Could you check a few things on this model? Use its own coordinates, in mm. Face numbers are marked on the shaded views. A direction names the side the tool comes from. Give positions to 0.01 mm unless a question says otherwise; leave off trailing zeros. Order: outer loops, then holes, each group sorted by start corner. A loop starts at its lowest first (then second) coordinate and runs counter-clockwise, first axis right, second up.
from build123d import *

# Parameters (mm, degrees)
F2_SIZE = 5
F3_SIZE = 3
F4_SIZE = 1


with BuildPart() as f1:
    # F0 (on Front) → F1 (revolve)
    with BuildSketch(Plane.XZ):
        Polygon((0, 5), (0, 0), (55, 0), (55, 12), (26, 12), (26, 19.5), (4, 19.5), (4, 7.25), (-2, 7.25), (-2, 5), align=None)
    revolve(axis=Axis((27.5, 0, 0), (-1, 0, 0)))

    # F2
    f2_edges = [f1.edges().sort_by_distance(p)[0] for p in [
        (4, 0, -19.5),
    ]]
    chamfer(f2_edges, length=F2_SIZE)

    # F3
    f3_edges = [f1.edges().sort_by_distance(p)[0] for p in [
        (26, 0, -19.5),
        (55, 0, -12),
    ]]
    chamfer(f3_edges, length=F3_SIZE)

    # F4
    f4_edges = [f1.edges().sort_by_distance(p)[0] for p in [
        (-2, 0, -7.25),
    ]]
    chamfer(f4_edges, length=F4_SIZE)


solid = f1.part
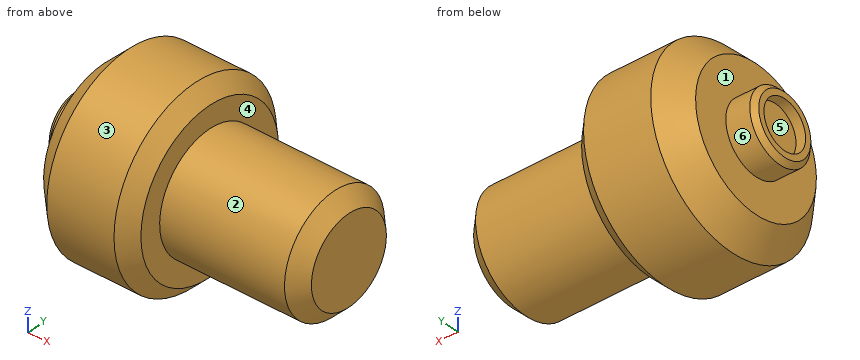
Item 1: For pin 1 (5 mm diameter, centred on y = 0, z = -1.5, fed in from -X); pin 2 (1.5 mm diameter, centred on x = 30, z = 11.5, fed in from -Y); pin 3 (1.5 mm diameter, centred on y = -6.5, z = 15.5, fed in from +X), each with a flat end and sliding along its axis, tell me the tip position at first contact or that it passes through.
Findings:
pin 1: stops at x = 0
pin 2: stops at y = -5.33
pin 3: stops at x = 26
Item 2: Imagine slicing it at A-A on y = 0. List the corners of the cut face in (x, z) for me, then the cut area to 3 significant figures.
Findings:
outline: (-2, -6.25) - (-1, -7.25) - (4, -7.25) - (4, -14.5) - (9, -19.5) - (23, -19.5) - (26, -16.5) - (26, -12) - (52, -12) - (55, -9) - (55, 9) - (52, 12) - (26, 12) - (26, 16.5) - (23, 19.5) - (9, 19.5) - (4, 14.5) - (4, 7.25) - (-1, 7.25) - (-2, 6.25) - (-2, 5) - (0, 5) - (0, -5) - (-2, -5) - close
area: 1,580 mm2
Item 3: Please list where these lines run through material, in increasing order: line 1 along Y through (x, z) = (18.5, 0); line 2 along Y through (x, z) = (-1, 0); line 3 along X through (y, z) = (-3, 12.5).
Findings:
line 1: y = -19.5 to 19.5
line 2: y = -7.25 to -5, 5 to 7.25
line 3: x = 4 to 26
Item 4: Imagine slicing it at C-C on x = 41. List the corners of the cut face in (y, z) for me.
Findings:
outline: circle Ø24 at (0, 0)
Item 5: For the marked faces 1, 2 and 3, which set-ups out of +Z, -Z, +X, -X, +Y, -Y let a thin tool reach every point of the face, with its end or its side?
Findings:
face 1: -X
face 2: +X
face 3: +X, -X
Item 6: Imagine slicing it at D-D on x = 20. List the corners of the cut face in (y, z) for me.
Findings:
outline: circle Ø39 at (0, 0)
Item 7: We'd pull the mould along Y, two halves only. Please class the marked faces 4, 5 and 6: +Y half, -Y half, draft (parallel to the pull), parting line (faces both ways), or undercut.
Findings:
face 4: draft
face 5: undercut
face 6: parting line
